from build123d import *

# Parameters (mm, degrees)
SKETCH1_R           = 2.1
BOSS_EXTRUDE1_DEPTH = 457
SKETCH19_R          = 2.1
BOSS_EXTRUDE7_DEPTH = 6
TAPPED_HOLE6_D      = 2.5
TAPPED_HOLE6_DEPTH  = 6


with BuildPart() as part:
    # Sketch1 → Boss-Extrude1 (new body)
    with BuildSketch(Plane(origin=(0, 0, 0), x_dir=(0, 0, -1), z_dir=(1, 0, 0))):
        with BuildLine():
            Line((-10, 9), (-10, 3))
            Line((-10, 3), (-8, 3))
            Line((-8, 3), (-8, 6))
            Line((-8, 6), (-7.060660172, 6))
            Line((-7.060660172, 6), (-4, 2.939339828))
            Line((-4, 2.939339828), (-4, -2.939339828))
            Line((-4, -2.939339828), (-7.060660172, -6))
            Line((-7.060660172, -6), (-8, -6))
            Line((-8, -6), (-8, -3))
            Line((-8, -3), (-10, -3))
            Line((-10, -3), (-10, -9))
            ThreePointArc((-10, -9), (-9.707106781, -9.707106781), (-9, -10))
            Line((-9, -10), (9, -10))
            ThreePointArc((9, -10), (9.707106781, -9.707106781), (10, -9))
            Line((10, -9), (10, -3))
            Line((10, -3), (8, -3))
            Line((8, -3), (8, -6))
            Line((8, -6), (7.060660172, -6))
            Line((7.060660172, -6), (4, -2.939339828))
            Line((4, -2.939339828), (4, 2.939339828))
            Line((4, 2.939339828), (7.060660172, 6))
            Line((7.060660172, 6), (8, 6))
            Line((8, 6), (8, 3))
            Line((8, 3), (10, 3))
            Line((10, 3), (10, 9))
            ThreePointArc((10, 9), (9.707106781, 9.707106781), (9, 10))
            Line((9, 10), (3, 10))
            Line((3, 10), (3, 8))
            Line((3, 8), (6, 8))
            Line((6, 8), (6, 7.060660172))
            Line((6, 7.060660172), (2.939339828, 4))
            Line((2.939339828, 4), (-2.939339828, 4))
            Line((-2.939339828, 4), (-6, 7.060660172))
            Line((-6, 7.060660172), (-6, 8))
            Line((-6, 8), (-3, 8))
            Line((-3, 8), (-3, 10))
            Line((-3, 10), (-9, 10))
            ThreePointArc((-9, 10), (-9.707106781, 9.707106781), (-10, 9))
        make_face()
        Circle(SKETCH1_R, mode=Mode.SUBTRACT)
        with BuildLine():
            Line((-6, -7.267766953), (-6, -7.5))
            ThreePointArc((-6, -7.5), (-5.853553391, -7.853553391), (-5.5, -8))
            Line((-5.5, -8), (5.5, -8))
            ThreePointArc((5.5, -8), (5.853553391, -7.853553391), (6, -7.5))
            Line((6, -7.5), (6, -7.267766953))
            ThreePointArc((6, -7.267766953), (5.961939766, -7.076425237), (5.853553391, -6.914213562))
            Line((5.853553391, -6.914213562), (3.085786438, -4.146446609))
            ThreePointArc((3.085786438, -4.146446609), (2.923574763, -4.038060234), (2.732233047, -4))
            Line((2.732233047, -4), (-2.732233047, -4))
            ThreePointArc((-2.732233047, -4), (-2.923574763, -4.038060234), (-3.085786438, -4.146446609))
            Line((-3.085786438, -4.146446609), (-5.853553391, -6.914213562))
            ThreePointArc((-5.853553391, -6.914213562), (-5.961939766, -7.076425237), (-6, -7.267766953))
        make_face(mode=Mode.SUBTRACT)
    extrude(amount=BOSS_EXTRUDE1_DEPTH)

    # Sketch19 → Boss-Extrude7 (add)
    with BuildSketch(Plane(origin=(457, 0, 0), x_dir=(0, 0, -1), z_dir=(1, 0, 0))):
        Circle(SKETCH19_R)
    extrude(amount=-BOSS_EXTRUDE7_DEPTH)

    # Tapped Hole6
    with Locations(Plane(origin=(457, 0, -33.955827028), x_dir=(0, 0, 1), z_dir=(1, 0, 0))):
        with Locations((33.955827028, 0)):
            Hole(TAPPED_HOLE6_D / 2, depth=TAPPED_HOLE6_DEPTH)


solid = part.part
The model under review builds one solid part; all positions refer to its coordinate system, in mm. Round coordinates to 2 decimals unless told otherwise and drop trailing zeros. Write item = value, one per line. Start each with the question number.
Item 1: For line 1 along Y through (x, z) = (343, 0); line 2 along Y through (x, z) = (423.5, -0.5); line 3 along Z through (x, y) = (123, -6.5), list the stretches that pass through material, from the lowest coordinate up.
Item 2: Mouldability with a two-part tool opening along Z and no side actions: class faces 1 (the face through (225, -8, 0)), 2 (the face through (457, -2, 0)) as released by +Z, released by -Z, zero draft, split by the parting line, or undercut.
Item 3: Clearance check with flat-ended pins moving along their axes: pin 1 Ø0.6 at (x, y) = (196, 9.5) entering from +Z; pin 2 Ø0.6 at (x, y) = (212.5, 9.5) entering from -Z; pin 3 Ø1.8 at (x, y) = (180.5, 0.5) entering from +Z. State where each tip first meets the part, or that it passes through.
Item 4: Consider section A-A on x = 38.5. Count the separate pieces of the cut face and the enclosed holes in it, plus the area to 3 significant figures.
Conclusion:
q1.line_1 = -10 to -8, -4 to -2.1, 2.1 to 4
q1.line_2 = -10 to -8, -4 to -2.04, 2.04 to 4
q1.line_3 = -10 to -5.44, 5.44 to 10
q2.face_1 = undercut
q2.face_2 = zero draft
q3.pin_1 = 9.98
q3.pin_2 = -9.98
q3.pin_3 = 4
q4.separate_pieces = 1
q4.enclosed_holes = 2
q4.area = 195 mm2
